Geometry check sheet. Reference: the model listing, model coordinates, mm. Give positions to 0.01 mm unless a question says otherwise; leave off trailing zeros. Write each loop counter-clockwise with the first axis right and the second up, starting at its lowest first coordinate (ties: lowest second). Pieces come first, ordered by that corner, then holes. Notation, with made-up numbers: (-8.75, 48) -> (47.25, 48) arc R20 cw to (47.25, 55) -> close; hole circle Ø7 at (-3.75, -21). An arc over 180 degrees is marked (long way). One line per item, written item: value.
from build123d import *

# Parameters (mm, degrees)
F0_R     = 8.255
F0_R_2   = 7.62
F1_DEPTH = 38.1
F2_R     = 9.04875
F2_R_2   = 8.255
F2_R_3   = 7.62
F3_DEPTH = 1.27
F4_R     = 0.508


with BuildPart() as f1:
    # F0 (on Front) → F1 (new body)
    with BuildSketch(Plane.XZ):
        Circle(F0_R)
        Circle(F0_R_2, mode=Mode.SUBTRACT)
    extrude(amount=F1_DEPTH)

    # F2 (on face) → F3 (join)
    with BuildSketch(Plane.XZ.offset(38.1)):
        Circle(F2_R)
        Circle(F2_R_2, mode=Mode.SUBTRACT)
        Circle(F2_R_2)
        Circle(F2_R_3, mode=Mode.SUBTRACT)
    extrude(amount=F3_DEPTH)

    # F4
    f4_edges = [f1.edges().sort_by_distance(p)[0] for p in [
        (-9.04875, -38.1, 0),
    ]]
    fillet(f4_edges, radius=F4_R)


solid = f1.part
1) Scan lines: probe 1 along Z at (x, y) = (0, -25) (3 decimals); probe 2 along Z at (x, y) = (-6, -16.5); probe 3 along X at (y, z) = (-2, 5.5). Record each from-to range of solid material in increasing order.
Verdict:
probe 1: -8.255 to -7.62, 7.62 to 8.255
probe 2: -5.67 to -4.7, 4.7 to 5.67
probe 3: -6.16 to -5.27, 5.27 to 6.16
2) Mould release check, pull along X, two halves, no side actions. Record for faces 1 (the flat face through (5.5, 0, -5.5)), 2 (the cylindrical face through (7.874, -18.783, 2.48)), 3 (the cylindrical face through (-1.65, -19.41, -7.44)): released by +X, released by -X, zero draft, split by the parting line, or undercut.
Verdict:
face 1: zero draft
face 2: split by the parting line
face 3: undercut
3) Sectioned sample at A-A on z = 0. Record the cut outline in (x, y) (3 decimals), plus the area to 3 significant figures.
Verdict:
outline: (-9.049, -39.37) -> (-7.62, -39.37) -> (-7.62, 0) -> (-8.255, 0) -> (-8.255, -38.1) -> (-8.541, -38.1) arc R0.508 ccw to (-9.049, -38.608) -> close; (7.62, -39.37) -> (9.049, -39.37) -> (9.049, -38.608) arc R0.508 ccw to (8.541, -38.1) -> (8.255, -38.1) -> (8.255, 0) -> (7.62, 0) -> close
area: 51.9 mm^2
4) Depth check by flat-ended pin: pin 1 Ø5 at (y, z) = (-11, -4.5) entering from +X; pin 2 Ø3 at (y, z) = (-31.5, -4.5) entering from -X; pin 3 Ø4 at (y, z) = (-29, -1) entering from +X (3 decimals). Enter the tip coordinate at first touch or a pass-through.
Verdict:
pin 1: x = 8.01
pin 2: x = -7.69
pin 3: x = 8.255
5) Sectioned sample at B-B on x = 0. Record the cut outline in (y, z) (3 decimals).
Verdict:
outline: (-39.37, -9.049) -> (-38.608, -9.049) arc R0.508 ccw to (-38.1, -8.541) -> (-38.1, -8.255) -> (0, -8.255) -> (0, -7.62) -> (-39.37, -7.62) -> close; (-39.37, 7.62) -> (0, 7.62) -> (0, 8.255) -> (-38.1, 8.255) -> (-38.1, 8.541) arc R0.508 ccw to (-38.608, 9.049) -> (-39.37, 9.049) -> close
6) Sectioned sample at C-C on y = -20. Record the cut outline in (x, z) (3 decimals), plus the area to 3 significant figures.
Verdict:
outline: circle Ø16.51 at (0, 0); hole circle Ø15.24 at (0, 0)
area: 31.7 mm^2
